Read the model definition and answer for the solid it produces. Units are mm, in the model's axes. A direction names the side the tool comes from. Coordinates: 2 decimals unless noted, no trailing zeros. Order: outer loops, then holes, each group sorted by start corner. A loop starts at its lowest first (then second) coordinate and runs counter-clockwise, first axis right, second up. Notation, with made-up numbers: M -9.5,-10 L 13.5,-10 A14 cw 13.5,10 Z; hole C -36.5,51 d4. An arc over 180 degrees is marked long. One line per question, with ' | ' between items. Start each with the question number.
1) Find section D-D, the plane x = -4.75. Write down the section's boundary in (y, z), plus the area to 3 significant figures.
2) A tool of negligible diameter and unlimited length cuts with its end or side. For faces 1 (the face through (-3, 4.7, -3)), 2 (the face through (0, 2, -6)), from which of +Z, -Z, +X, -X, +Y, -Y can it reach the whole face along a straight path? Write none if from no direction.
3) Consider probe 1 along Y at (x, z) = (0, 4.5); probe 2 along Y at (x, z) = (-3.5, -1.5); probe 3 along X at (y, z) = (2.5, 5.5). Determine where each line is inside the solid, lowest interval first.
4) Given P1, Ø3, axis at y = 3, z = -4, coming from the +X side; P2, Ø3, axis at x = -4, z = 3.5, coming from the +Y side, each flat-ended and moving along its own axis, determine where each tip first touches the part or whether it passes through.
5) Find section A-A, the plane y = 4. Write down the section's boundary in (x, z), plus the area to 3 significant figures.
6) Find section C-C, the plane y = 7.5. Write down the section's boundary in (x, z).
7) Find section B-B, the plane x = -3.25. Write down the section's boundary in (y, z), plus the area to 3 significant figures.
from build123d import *

# Parameters (mm, degrees)
BOSS_EXTRUDE1_DEPTH = 4.7
SKETCH2_R           = 4
BOSS_EXTRUDE2_DEPTH = 2.2
SKETCH3_R           = 2.7
BOSS_EXTRUDE3_DEPTH = 2.7
FILLET1_R           = 1.5


with BuildPart() as part:
    # Sketch1 → Boss-Extrude1 (new body)
    with BuildSketch(Plane(origin=(0, 0, 0), x_dir=(1, 0, 0), z_dir=(0, 1, 0))):
        with BuildLine():
            Line((-3.60441458, 6), (3.60558542, 6))
            ThreePointArc((3.60558542, 6), (7.00058542, 0), (3.60558542, -6))
            Line((3.60558542, -6), (-3.60441458, -6))
            ThreePointArc((-3.60441458, -6), (-6.99941458, 0), (-3.60441458, 6))
        make_face()
    extrude(amount=BOSS_EXTRUDE1_DEPTH)

    # Sketch2 → Boss-Extrude2 (add)
    with BuildSketch(Plane(origin=(0, 4.7, 0), x_dir=(1, 0, 0), z_dir=(0, 1, 0))):
        with Locations(Location((0, 0, 0), (0, 0, 270))):
            Circle(SKETCH2_R)
    extrude(amount=BOSS_EXTRUDE2_DEPTH)

    # Sketch3 → Boss-Extrude3 (add)
    with BuildSketch(Plane(origin=(0, 6.9, 0), x_dir=(1, 0, 0), z_dir=(0, 1, 0))):
        with Locations(Location((0, 0, 0), (0, 0, 270))):
            Circle(SKETCH3_R)
    extrude(amount=BOSS_EXTRUDE3_DEPTH)

    # Fillet1
    fillet1_edges = [part.edges().sort_by_distance(p)[0] for p in [
        (0, 9.6, -2.7),
    ]]
    fillet(fillet1_edges, radius=FILLET1_R)


solid = part.part
Report:
1) outline: M 0,-5.14 L 4.7,-5.14 L 4.7,5.14 L 0,5.14 Z | area: 48.3 mm^2
2) face 1: +Y | face 2: -Z, +X, -X, +Y, -Y
3) probe 1: y = 0 to 4.7 | probe 2: y = 0 to 6.9 | probe 3: x = -4.33 to 4.33
4) P1: stops at x = 6.54 | P2: stops at y = 6.9
5) outline: M -3.6,-6 L 3.61,-6 A7 ccw 3.61,6 L -3.6,6 A7 ccw Z | area: 144 mm^2
6) outline: C 0,0 d5.4
7) outline: M 0,-6 L 4.7,-6 L 4.7,-2.33 L 6.9,-2.33 L 6.9,2.33 L 4.7,2.33 L 4.7,6 L 0,6 Z | area: 66.7 mm^2
